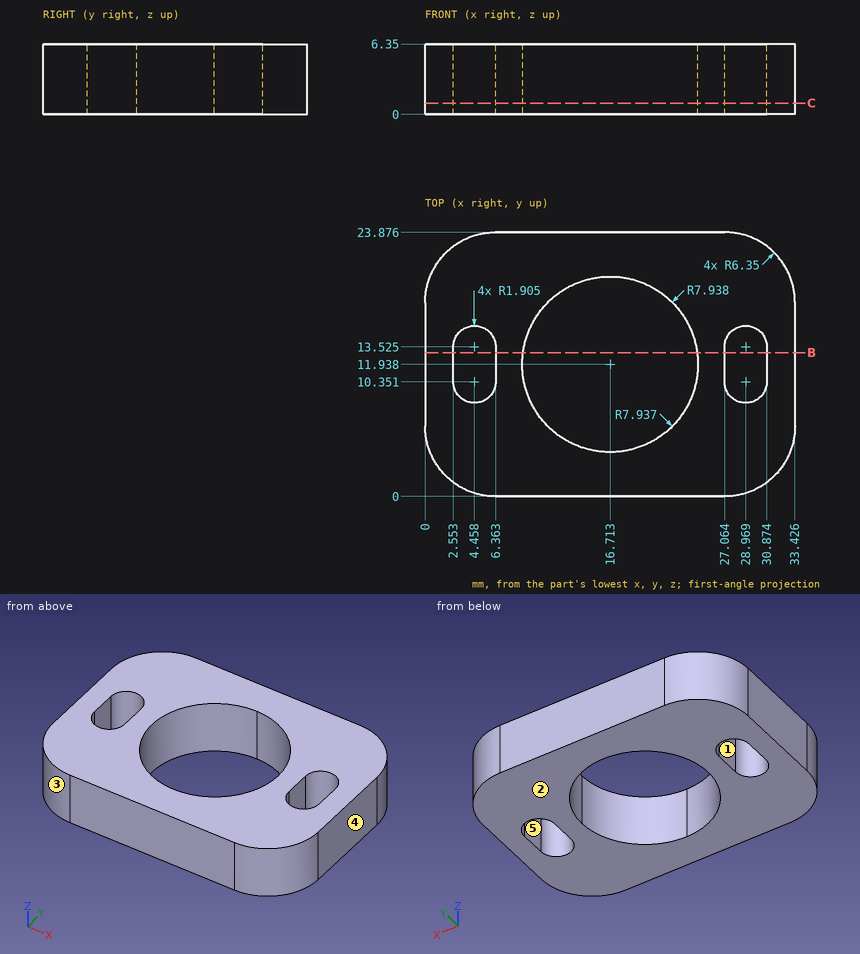
Check sheet for the drawn part. Datum: minimum x, y, z corner. Units: mm. A direction names the side the tool comes from. Round coordinates to 2 decimals unless told otherwise and drop trailing zeros. Loops run counter-clockwise (first coordinate to the right, second up) from the corner with the lowest first, then second, coordinate; pieces in that order, holes last. Notation, with made-up numbers: (36.25, -40) -> (64.25, -40) arc R29 cw to (64.25, -19) -> close; hole circle Ø3 at (7, 20.25). An arc over 180 degrees is marked (long way). Put each result on its own line as item: value. Start each with the question number.
1. Draft check along Y on the marked faces 1, 2 and 3. Enter one of: +Y half, -Y half, draft (parallel to the pull), parting line (faces both ways), or undercut.
2. Scan lines: probe 1 along X at (y, z) = (14.25, 6) (1 decimal); probe 2 along X at (y, z) = (12.5, 2) (1 decimal); probe 3 along X at (y, z) = (7.25, 4) (1 decimal). Record each from-to range of solid material in increasing order.
3. Gauge pin test, flat end, axial feed: pin 1 (10 mm diameter, centred on x = 8.5, y = 20, fed in from -Z). Record the tip position at first contact, or that the pin passes through.
4. Section check C-C (z = 1). Give the number of separate pieces and of enclosed holes in the cut face.
5. Access from +Z, -Z, +X, -X, +Y, -Y to the whole of each face (thin tool, end or side, straight path). Record for the marked faces 4 and 5.
6. Section check B-B (y = 13). Enter the section's corners in (x, z).
Findings:
1. face 1: undercut
1. face 2: draft
1. face 3: -Y half
2. probe 1: x = 0 to 2.7, 6.2 to 9.1, 24.3 to 27.2, 30.7 to 33.4
2. probe 2: x = 0 to 2.6, 6.4 to 8.8, 24.6 to 27.1, 30.9 to 33.4
2. probe 3: x = 0 to 10.3, 23.1 to 33.4
3. pin 1: stops at z = 0
4. separate pieces: 1
4. enclosed holes: 3
5. face 4: +Z, -Z, +X, +Y, -Y
5. face 5: +Z, -Z
6. outline: (0, 0) -> (2.55, 0) -> (2.55, 6.35) -> (0, 6.35) -> close; (6.36, 0) -> (8.85, 0) -> (8.85, 6.35) -> (6.36, 6.35) -> close; (24.58, 0) -> (27.06, 0) -> (27.06, 6.35) -> (24.58, 6.35) -> close; (30.87, 0) -> (33.43, 0) -> (33.43, 6.35) -> (30.87, 6.35) -> close
